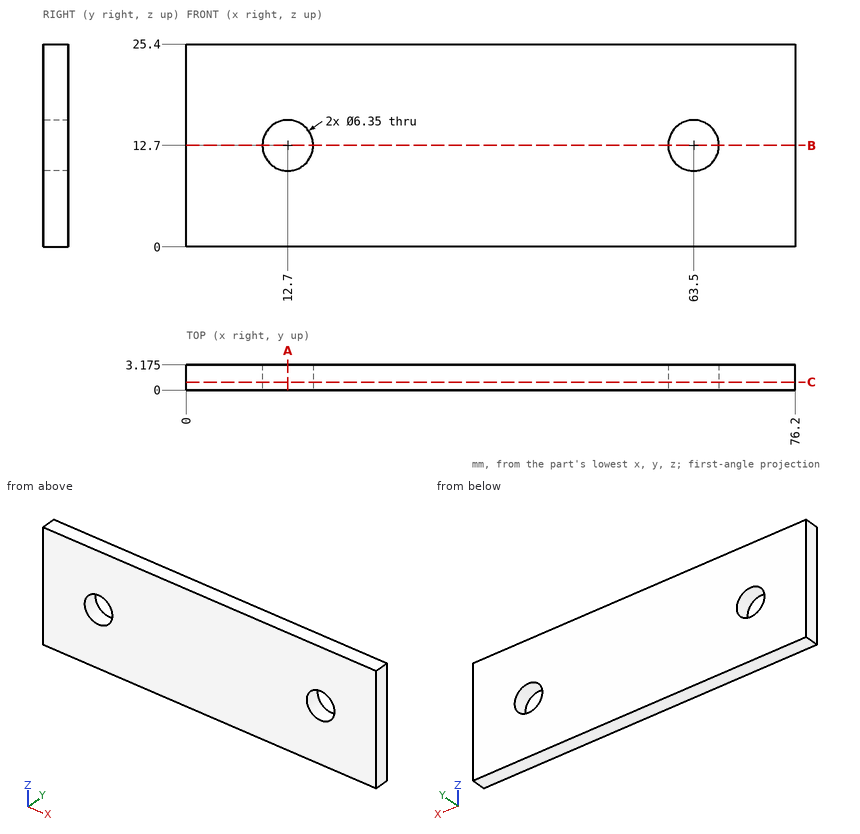
Drawing for the job (mm, zero at the part's lowest x, y, z). Give positions to 0.01 mm unless a question says otherwise; leave off trailing zeros. Write each loop counter-clockwise with the first axis right and the second up, starting at its lowest first coordinate (ties: lowest second). Pieces come first, ordered by that corner, then holes. Notation, with made-up numbers: (28, 69) - (32, 69) arc R20 ccw to (32, 100) - close; hole circle Ø8 at (13, 52.5). An arc over 180 degrees is marked (long way). Answer as CSV lines item,"result".
Q1. Band-saw the part on C-C (y = 1). Give the cut face in (x, z) (3 decimals).
Result set:
outline,"(0, 0) - (76.2, 0) - (76.2, 25.4) - (0, 25.4) - close; hole circle Ø6.35 at (12.7, 12.7); hole circle Ø6.35 at (63.5, 12.7)"
Q2. Drill centre lines: line 1 (X direction, y = 2.2, z = 12.7) (3 decimals); line 2 (Z direction, x = 63.5, y = 2.45) (3 decimals); line 3 (Z direction, x = 14, y = 2.8). Where is each one in solid material? Low to high. Write a range as from..to.
Result set:
line 1,"0..9.525, 15.875..60.325, 66.675..76.2"
line 2,"0..9.525, 15.875..25.4"
line 3,"0..9.8, 15.6..25.4"
Q3. Band-saw the part on A-A (x = 12.7). Give the cut face in (y, z) (3 decimals), and give its area (3 significant figures).
Result set:
outline,"(0, 0) - (3.175, 0) - (3.175, 9.525) - (0, 9.525) - close; (0, 15.875) - (3.175, 15.875) - (3.175, 25.4) - (0, 25.4) - close"
area,"60.5 mm²"
Q4. Flat gauge pin, fed straight in: pin 1 Ø5 at (x, z) = (12.7, 12.7) entering from +Y. Where does the tip first touch, or does it go through?
Result set:
pin 1,"through"
Q5. Band-saw the part on B-B (z = 12.7). Give the cut face in (x, y) (3 decimals), and give its area (3 significant figures).
Result set:
outline,"(0, 0) - (9.525, 0) - (9.525, 3.175) - (0, 3.175) - close; (15.875, 0) - (60.325, 0) - (60.325, 3.175) - (15.875, 3.175) - close; (66.675, 0) - (76.2, 0) - (76.2, 3.175) - (66.675, 3.175) - close"
area,"202 mm²"
